Autodesk Inventor part; units mm, degrees
ref_plane "YZ Plane" through (0, 0, 0) normal (1, 0, 0) x (0, 1, 0)
ref_plane "XZ Plane" through (0, 0, 0) normal (0, 1, 0) x (-1, 0, 0)
ref_plane "XY Plane" through (0, 0, 0) normal (0, 0, 1) x (1, 0, 0)
sketch "Sketch1" plane through (0, 0, 0) normal (1, 0, 0) x (0, 1, 0)
  circle A0 centre (0, 0) radius 150
  dimension "d0" = 300
extrude "Extrusion1" add sketch "Sketch1" along normal blind 42
sketch "Sketch2" plane through (42, 0, 0) normal (1, 0, 0) x (0, 0, -1)
  circle A0 centre (0, 0) radius 140
  dimension "d3" = 280
extrude "Extrusion2" add sketch "Sketch2" along normal blind 312
sketch "Sketch3" plane through (354, 0, 0) normal (1, 0, 0) x (0, 0, -1)
  circle A0 centre (0, 0) radius 100
  dimension "d6" = 200
extrude "Extrusion3" add sketch "Sketch3" along normal blind 188
chamfer "Chamfer1" distance 5 angle 15 1 edges at (354, 0, 140) measured on face at (354, 2.3252, 126.4215)
chamfer "Chamfer2" distance 3 angle 45 1 edges at (542, 0, 100) measured on face at (542, 30.5098, 9.4965)
fillet "Fillet1" radius 15 1 edges at (354, 0, 100)
properties part number "eje"
Input: part model. Units: mm. Frame: model coordinates. A direction names the side the tool comes from. Round coordinates to 2 decimals unless told otherwise and drop trailing zeros. Loops run counter-clockwise (first coordinate to the right, second up) from the corner with the lowest first, then second, coordinate; pieces in that order, holes last.
1) Section query A-A on y = 0. Return the cut outline in (x, z), plus the area to 3 significant figures.
Ans:
outline: (0, -150) - (42, -150) - (42, -140) - (352.66, -140) - (354, -135) - (354, -115) arc R15 cw to (369, -100) - (539, -100) - (542, -97) - (542, 97) - (539, 100) - (369, 100) arc R15 cw to (354, 115) - (354, 135) - (352.66, 140) - (42, 140) - (42, 150) - (0, 150) - close
area: 138,000 mm2
2) Set-up query: faces 1 (the cylindrical face through (452.81, -30.04, -95.38)), 2 (the flat face through (542, 1, 1)). Return all of +Z, -Z, +X, -X, +Y, -Y with unobstructed straight access to the full face (end or side cutting, diameter ignored); none if empty.
Ans:
face 1: +X
face 2: +Z, -Z, +X, +Y, -Y
3) Material intervals for line 1 (X direction, y = -113.5, z = -72.5); line 2 (X direction, y = 113.5, z = 3.5); line 3 (Y direction, x = 474, z = 1.5), sorted ascending.
Ans:
line 1: x = 0 to 354
line 2: x = 0 to 354.07
line 3: y = -99.99 to 99.99
4) Section query C-C on x = 109. Return the cut outline in (y, z), plus the area to 3 significant figures.
Ans:
outline: circle Ø280 at (0, 0)
area: 61,600 mm2
5) Pin query (flat end, axial travel): pin 1 (8 mm diameter, centred on y = -51, z = -90, fed in from -X); pin 2 (8 mm diameter, centred on x = 217, y = 101.5, fed in from -Z); pin 3 (6 mm diameter, centred on x = 398, y = 91.5, fed in from -Z); pin 4 (3 mm diameter, centred on x = 445.5, z = 88, fed in from -Y). Return the tip coordinate at first contact, or that it passes through.
Ans:
pin 1: stops at x = 0
pin 2: stops at z = -100.47
pin 3: stops at z = -46.56
pin 4: stops at y = -50.18
